Read the model definition and answer for the solid it produces. Units are mm, in the model's axes. A direction names the side the tool comes from. Coordinates: 2 decimals unless noted, no trailing zeros. Write each loop counter-clockwise with the first axis right and the second up, starting at its lowest first coordinate (ties: lowest second). Pieces come first, ordered by that corner, then holes.
from build123d import *

# Parameters (mm, degrees)
CROQUIS2_R                   = 5
SALIENTE_EXTRUIR1_DEPTH      = 22
CROQUIS3_R                   = 10
CROQUIS3_W                   = 50
CROQUIS3_H                   = 69
CORTAR_EXTRUIR1_DEPTH        = 8
CROQUIS4_R                   = 10
CORTAR_EXTRUIR2_DEPTH        = 8
CROQUIS5_W                   = 14.5
CROQUIS5_H                   = 64
SALIENTE_EXTRUIR2_REACH      = 203.856
SALIENTE_EXTRUIR2_END_RADIUS = 32
CROQUIS9_W                   = 45
CROQUIS9_H                   = 40
SALIENTE_EXTRUIR3_DEPTH      = 25
CROQUIS10_W                  = 45
CROQUIS10_H                  = 10


with BuildPart() as part:
    # Croquis2 → Saliente-Extruir1 (new body)
    with BuildSketch(Plane(origin=(0, 0, 0), x_dir=(1, 0, 0), z_dir=(0, 1, 0))):
        with BuildLine():
            Line((20, 0), (140, 0))
            ThreePointArc((140, 0), (154.142135624, 5.857864376), (160, 20))
            Line((160, 20), (160, 89))
            Line((160, 89), (0, 89))
            Line((0, 89), (0, 20))
            ThreePointArc((0, 20), (5.857864376, 5.857864376), (20, 0))
        make_face()
        with Locations(Location((20, 20, 0), (0, 0, 270))):
            Circle(CROQUIS2_R, mode=Mode.SUBTRACT)
        with Locations(Location((140, 20, 0), (0, 0, 270))):
            Circle(CROQUIS2_R, mode=Mode.SUBTRACT)
        with Locations(Location((80, 55, 0), (0, 0, 270))):
            Circle(CROQUIS2_R, mode=Mode.SUBTRACT)
    extrude(amount=SALIENTE_EXTRUIR1_DEPTH)

    # Croquis3 → Cortar-Extruir1 (cut)
    with BuildSketch(Plane(origin=(0, 22, 0), x_dir=(1, 0, 0), z_dir=(0, 1, 0))):
        with Locations(Location((20, 20, 0), (0, 0, 270))):
            Circle(CROQUIS3_R)
        with Locations(Location((140, 20, 0), (0, 0, 270))):
            Circle(CROQUIS3_R)
        with Locations((80, 34.5)):
            Rectangle(CROQUIS3_W, CROQUIS3_H)
    extrude(amount=-CORTAR_EXTRUIR1_DEPTH, mode=Mode.SUBTRACT)

    # Croquis4 → Cortar-Extruir2 (cut)
    with BuildSketch(Plane(origin=(0, 14, 0), x_dir=(1, 0, 0), z_dir=(0, 1, 0))):
        with Locations(Location((80, 55, 0), (0, 0, 270))):
            Circle(CROQUIS4_R)
    extrude(amount=-CORTAR_EXTRUIR2_DEPTH, mode=Mode.SUBTRACT)



with BuildPart() as body_2:
    # Croquis5 → Revolución1 (revolve)
    with BuildSketch(Plane(origin=(0, 75, 0), x_dir=(1, 0, 0), z_dir=(0, 1, 0)), mode=Mode.PRIVATE) as revoluci_n1_sk:
        with Locations((152.75, 57)):
            Rectangle(CROQUIS5_W, CROQUIS5_H)
    revolve(revoluci_n1_sk.sketch.rotate(Axis((128, 75, -107.397420406), (0, 0, 1)), 180), axis=Axis((128, 75, -107.397420406), (0, 0, 1)))


with BuildPart() as part_1:
    add(part.part)

    add(body_2.part)  # Saliente-Extruir2 merges body 2
    # Saliente-Extruir2: up to this cylinder (the profile starts outside it)
    saliente_extruir2_end = Plane(origin=(128, 75, -70.113997), z_dir=(0, 0, -1)) * Cylinder(SALIENTE_EXTRUIR2_END_RADIUS, 472.712, mode=Mode.PRIVATE)
    # Croquis8 → Saliente-Extruir2 (add, up to the surface)
    with BuildSketch(Plane(origin=(0, 22, 0), x_dir=(1, 0, 0), z_dir=(0, 1, 0)), mode=Mode.PRIVATE) as saliente_extruir2_sk1:
        with BuildLine():
            Line((96, 89), (96, 73))
            Line((96, 73), (120, 73))
            Line((120, 73), (120, 39))
            ThreePointArc((120, 39), (128, 31), (136, 39))
            Line((136, 39), (136, 73))
            Line((136, 73), (160, 73))
            Line((160, 73), (160, 89))
            Line((160, 89), (96, 89))
        make_face()
    saliente_extruir2_tool1 = extrude(saliente_extruir2_sk1.sketch, amount=SALIENTE_EXTRUIR2_REACH, mode=Mode.PRIVATE) - saliente_extruir2_end
    add(saliente_extruir2_tool1.solids().sort_by_distance((128, 22, -70.113997))[0])

    # Croquis9 → Saliente-Extruir3 (add)
    with BuildSketch(Plane(origin=(0, 22, 0), x_dir=(1, 0, 0), z_dir=(0, 1, 0))):
        with Locations((22.5, 53)):
            Rectangle(CROQUIS9_W, CROQUIS9_H)
    extrude(amount=SALIENTE_EXTRUIR3_DEPTH)

    # Croquis10 → Cortar-Revolución1 (revolve, cut)
    with BuildSketch(Plane(origin=(0, 47, 0), x_dir=(1, 0, 0), z_dir=(0, 1, 0))):
        with Locations((22.5, 58)):
            Rectangle(CROQUIS10_W, CROQUIS10_H)
    revolve(axis=Axis((45, 47, -53), (-1, 0, 0)), mode=Mode.SUBTRACT)


solid = part_1.part
Item 1: For faces 1 (the flat face through (45, 32, -53)), 2 (the flat face through (105, 18, -34)), 3 (the flat face through (22, 47, -68)), 4 (the flat face through (150, 36, -73)), 5 (the flat face through (55, 18, -34)), determine the directions among +Z, -Z, +X, -X, +Y, -Y from which every point of the face is accessible in a straight line to the end or side of a thin tool.
Item 2: The part is cut by section C-C (y = 29). Give the vertices of the cut face in (x, z), and give its area (3 significant figures).
Item 3: The part is cut by section B-B (x = 80). Give the vertices of the cut face in (y, z), and give its area (3 significant figures).
Item 4: Find the intervals of material crossed by probe 1 along X at (y, z) = (17, -20); probe 2 along Y at (x, z) = (128, -48); probe 3 along Y at (x, z) = (137, -68.5), in increasing order.
Item 5: The part is cut by section D-D (z = -23). Give the vertices of the cut face in (x, y).
Item 6: The part is cut by section A-A (z = -55). Give the vertices of the cut face in (x, y), and give its area (3 significant figures).
Item 7: Given pin 1 (7.5 mm diameter, centred on x = 29, y = 32, fed in from -Z); pin 2 (2 mm diameter, centred on y = 59.5, z = -22.5, fed in from +X); pin 3 (10 mm diameter, centred on x = 142, z = -17.5, fed in from +Y); pin 4 (8 mm diameter, centred on y = 81, z = -33.5, fed in from +X), each flat-ended and moving along its own axis, determine where each tip first touches the part or whether it passes through.
Item 8: Determine the mould class of faces 6 (the flat face through (145, 14, -18)), 7 (the flat face through (99, 41, -89)), 8 (the cylindrical face through (5.703, 10.846, -6.014)) for opening direction X: +X half, -X half, draft (parallel to the pull), parting line (faces both ways), or undercut.
Answer:
1. face 1: +Z, -Z, +Y
1. face 2: +Z
1. face 3: +Z, -Z, -X, +Y
1. face 4: +Z, +X
1. face 5: +Z, +Y
2. outline: (0, -73) - (45, -73) - (45, -33) - (0, -33) - close; (96, -89) - (160, -89) - (160, -73) - (136, -73) - (136, -39) arc R8 ccw to (120, -39) - (120, -73) - (96, -73) - close
2. area: 3,470 mm2
3. outline: (0, -89) - (22, -89) - (22, -69) - (14, -69) - (14, -65) - (6, -65) - (6, -60) - (0, -60) - close; (0, -50) - (6, -50) - (6, -45) - (14, -45) - (14, 0) - (0, 0) - close
3. area: 1,190 mm2
4. probe 1: x = 0 to 10, 30 to 55, 105 to 130, 150 to 160
4. probe 2: y = 0 to 57.5, 92.5 to 107
4. probe 3: y = 0 to 22, 44.29 to 59.99, 90.01 to 105.71
5. outline: (0, 0) - (16, 0) - (16, 14) - (10.46, 14) - (10.46, 22) - (0, 22) - close; (24, 0) - (136, 0) - (136, 14) - (130.46, 14) - (130.46, 22) - (105, 22) - (105, 14) - (55, 14) - (55, 22) - (29.54, 22) - (29.54, 14) - (24, 14) - close; (144, 0) - (160, 0) - (160, 22) - (149.54, 22) - (149.54, 14) - (144, 14) - close
6. outline: (0, 0) - (75, 0) - (75, 6) - (70, 6) - (70, 14) - (55, 14) - (55, 22) - (45, 22) - (45, 37.2) - (0, 37.2) - close; (85, 0) - (160, 0) - (160, 22) - (136, 22) - (136, 44.02) arc R32 ccw (long way) to (120, 44.02) - (120, 22) - (105, 22) - (105, 14) - (90, 14) - (90, 6) - (85, 6) - close; hole circle Ø35 at (128, 75)
6. area: 6,180 mm2
7. pin 1: stops at z = -73
7. pin 2: passes through
7. pin 3: stops at y = 14
7. pin 4: stops at x = 159.94
8. face 6: undercut
8. face 7: draft
8. face 8: -X half
